For this review, use the dimensioned drawing (mm, ordinates from the lowest corner) and the shaded views. Give positions to 0.01 mm unless a question says otherwise; leave off trailing zeros. Loops run counter-clockwise (first coordinate to the right, second up) from the corner with the lowest first, then second, coordinate; pieces in that order, holes last. Notation, with made-up numbers: M -9,36 L 16,36 A23 ccw 16,62 Z; hole C 53,-5 d6. An arc over 180 degrees is marked long. Return JSON: item names as keys, results as strings.
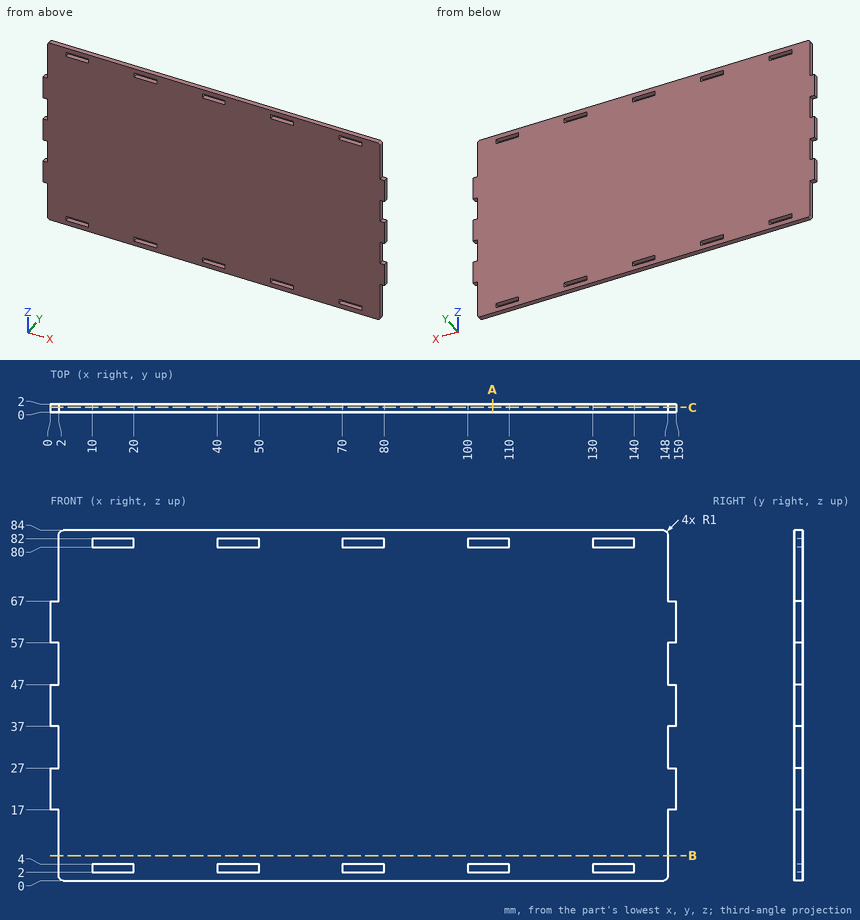
1) Insertion check: pin 1 (0.6 mm diameter, centred on y = 0.5, z = 81.5, fed in from +X); pin 2 (0.6 mm diameter, centred on y = 1, z = 81, fed in from -X). Each pin has a flat end and moves straight along its axis. Give the tip position at first contact, or say it passes through.
From the geometry:
{"pin 1": "x = 148", "pin 2": "x = 2"}
2) Wall thickness on L1, parallel to Z at x = 139, y = 1; L2, parallel to X at y = 0.6, z = 79: over which ranges is each line inside the solid? List them lowest first. Write a range as from..to.
From the geometry:
{"L1": "0..2, 4..80, 82..84", "L2": "2..148"}
3) Consider section A-A on x = 106. Write out the cut boundary in (y, z).
From the geometry:
{"outline": "M 0,0 L 2,0 L 2,2 L 0,2 Z; M 0,4 L 2,4 L 2,80 L 0,80 Z; M 0,82 L 2,82 L 2,84 L 0,84 Z"}
4) Consider section B-B on z = 6. Write out the cut boundary in (x, y).
From the geometry:
{"outline": "M 2,0 L 148,0 L 148,2 L 2,2 Z"}
5) Consider section C-C on y = 1.2. Count the separate pieces of the cut face and the enclosed holes in it, then the cut area to 3 significant figures.
From the geometry:
{"separate pieces": "1", "enclosed holes": "10", "area": "12,200 mm²"}
